For this review, take the finished solid that the model builds, in its own axes (mm). Face numbers are marked on the shaded views. A direction names the side the tool comes from. Coordinates: 2 decimals unless noted, no trailing zeros. Loops run counter-clockwise (first coordinate to the right, second up) from the corner with the lowest first, then second, coordinate; pieces in that order, holes last. Notation, with made-up numbers: M 25.25,-32 L 51.25,-32 A16 cw 51.25,-25 Z; hole C 43.25,17.5 d6. An arc over 180 degrees is marked long. Put each result on its own line as item: value.
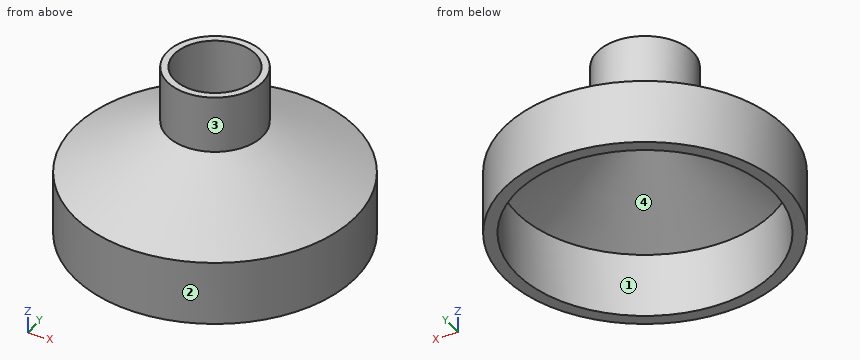
Autodesk Fusion 360 part; units mm, degrees
sketch "Boceto1" plane through (0, 0, 0) normal (0, 0, 1) x (1, 0, 0)
  circle A0 centre (0, 0) radius 39.5
  circle A1 centre (0, 0) radius 36
  dimension "d1" = 79
  dimension "d2" = -3.5
ref_plane "PlanoDeObra1" through (0, 0, 15) normal (0, 0, 1) x (1, 0, 0)
sketch "Boceto2" plane through (0, 0, 15) normal (0, 0, 1) x (1, 0, 0)
  circle A0 centre (0, 0) radius 13.375
  circle A1 centre (0, 0) radius 11.375
  dimension "d4" = 26.75
  dimension "d5" = -2
loft "Solevación1" add profiles "Boceto1", "Boceto2" section 1 section 2
loft "Solevación2" cut profiles "Boceto2", "Boceto1" section 1 contours A1 section 2 contours A1
extrude "Extruir1" add sketch "Boceto2" along normal blind 16
extrude "Extruir2" add sketch "Boceto1" against normal blind 18
(1) Add section C-C (z = 8.5). Write out the cut boundary in (x, y), plus the area to 3 significant figures.
Determined:
outline: C 0,0 d49.39; hole C 0,0 d44.09
area: 389 mm^2
(2) Add section A-A (x = 0). Write out the cut boundary in (y, z) (3 decimals).
Determined:
outline: M -39.5,-18 L -36,-18 L -36,0 L -11.375,15 L -11.375,31 L -13.375,31 L -13.375,15 L -39.5,0 Z; M 11.375,15 L 36,0 L 36,-18 L 39.5,-18 L 39.5,0 L 13.375,15 L 13.375,31 L 11.375,31 Z
(3) Add section B-B (z = -11.5). Write out the cut boundary in (x, y), plus the area to 3 significant figures.
Determined:
outline: C 0,0 d79; hole C 0,0 d72
area: 830 mm^2
(4) For pin 1 (12 mm diameter, centred on x = 1.5, y = -23, fed in from -Z); pin 2 (6 mm diameter, centred on y = 17.5, z = -8.5, fed in from +X); pin 3 (3 mm diameter, centred on x = 10, z = -4.5, fed in from -Y), all flat-tipped, find the tip position at first contact; note any pin that passes through.
Determined:
pin 1: stops at z = 4.23
pin 2: stops at x = 36.74
pin 3: stops at y = -38.57
(5) Wall thickness on line 1 along Y through (x, z) = (0, -5.5); line 2 along X through (y, z) = (-9.5, -13.5); line 3 along Y through (x, z) = (-12, -9.5): over which ranges is each line inside the solid? List them lowest first. Write a range as [from, to].
Determined:
line 1: y = [-39.5, -36], [36, 39.5]
line 2: x = [-38.34, -34.72], [34.72, 38.34]
line 3: y = [-37.63, -33.94], [33.94, 37.63]
(6) Tool access review of the marked faces 3 and 4: name each direction out of +Z, -Z, +X, -X, +Y, -Y from which nothing blocks a thin tool from reaching the whole face with its end or side.
Determined:
face 3: +Z
face 4: -Z
(7) Draft analysis for pull direction Y (two halves, no side actions). For the marked faces 1 and 2, state which applies: +Y half, -Y half, draft (parallel to the pull), parting line (faces both ways), or undercut.
Determined:
face 1: undercut
face 2: parting line
